Input: part model. Units: mm. Frame: model coordinates. A direction names the side the tool comes from. Give positions to 0.01 mm unless a question says otherwise; leave off trailing zeros. Order: outer loops, then holes, each group sorted by start corner. A loop starts at its lowest first (then second) coordinate and runs counter-clockwise, first axis right, second up. Notation, with made-up numbers: M -1,69 L 13,69 A9 ccw 13,77 Z; hole C 24.25,69 d6. An arc over 180 degrees is marked long. Use a Markdown table: item, result.
from build123d import *

# Parameters (mm, degrees)
F0_R     = 75
F0_R_2   = 67.5
F5_R     = 7.5
F6_DEPTH = 150


with BuildPart() as f2:
    # F2: sweep along a path in F1
    with BuildLine(Plane.XY) as f2_path:
        Line((0, 0), (0, 250))
        ThreePointArc((0, 250), (-41.0050506339, 348.9949493661), (-140, 390))
        Line((-140, 390), (-390, 390))
    # F0 (on Front) → F2 (sweep)
    with BuildSketch(Plane.XZ):
        Circle(F0_R)
        Circle(F0_R_2, mode=Mode.SUBTRACT)
    sweep(path=f2_path.line)

    # F5 (on face) → F6 (cut)
    with BuildSketch(Plane(origin=(267.132034356, 267.132034356, 0), x_dir=(-0.7071067812, 0.7071067812, 0), z_dir=(0.7071067812, 0.7071067812, 0))):
        with Locations((276.0982438922, 0)):
            Circle(F5_R)
    extrude(amount=-F6_DEPTH, mode=Mode.SUBTRACT)


solid = f2.part
1) Cut plane A-A on z = 22. Return loops of the section in (x, y).
Response values:
| item | result |
|---|---|
| outline | M -390,318.3 L -140,318.3 A68.3 cw -71.7,250 L -71.7,0 L -63.81,0 L -63.81,250 A76.19 ccw -140,326.19 L -390,326.19 Z; M -390,453.81 L -140,453.81 A203.81 cw 63.81,250 L 63.81,0 L 71.7,0 L 71.7,250 A211.7 ccw -140,461.7 L -390,461.7 Z |
2) First-contact query: pin 1 Ø2 at (x, z) = (-42.5, -37.5) entering from -Y; pin 2 Ø4 at (y, z) = (167.5, -53.5) entering from +X; pin 3 Ø2 at (y, z) = (144, -9) entering from +X. Flat tips, straight axial feed; report the tip coordinate or a pass-through.
Response values:
| item | result |
|---|---|
| pin 1 | stops at y = 419.2 |
| pin 2 | stops at x = 54.52 |
| pin 3 | stops at x = 74.57 |
3) Material intervals for line 1 (Z direction, x = -216, y = 390); line 2 (Y direction, x = -325, z = 0), sorted ascending. Write a range as from..to.
Response values:
| item | result |
|---|---|
| line 1 | z = -75..-67.5, 67.5..75 |
| line 2 | y = 315..322.5, 457.5..465 |
4) Cut plane C-C on z = -45. Return loops of the section in (x, y), and give its area (3 significant figures).
Response values:
| item | result |
|---|---|
| outline | M -390,330 L -140,330 A80 cw -60,250 L -60,0 L -50.31,0 L -50.31,250 A89.69 ccw -140,339.69 L -390,339.69 Z; M -390,440.31 L -140,440.31 A190.31 cw 50.31,250 L 50.31,0 L 60,0 L 60,250 A200 ccw -140,450 L -390,450 Z |
| area | 13,900 mm² |
5) Reachability of faces 1 (the face through (-266.75, 322.565, -2.968)), 2 (the face through (11, 0, 67)), 3 (the face through (-9.764, 126.75, -74.362)) from +Z, -Z, +X, -X, +Y, -Y: full face, straight path, thin tool, end or side. Return the list, or none.
Response values:
| item | result |
|---|---|
| face 1 | -X |
| face 2 | +Z, -Z, +X, -X, -Y |
| face 3 | -Y |
6) Mould query, pull axis Z, two halves, no side actions, for faces 4 (the face through (-390, 379, -67)), 5 (the face through (-266.75, 459.28, 28.73)), 6 (the face through (14.292, 394.157, 0.33)), 7 (the face through (-53.57, 126.75, 41.07)). Classes: released by +Z, released by -Z, zero draft, split by the parting line, or undercut.
Response values:
| item | result |
|---|---|
| face 4 | zero draft |
| face 5 | split by the parting line |
| face 6 | undercut |
| face 7 | undercut |
7) Cut plane B-B on x = -152. Return loops of the section in (y, z).
Response values:
| item | result |
|---|---|
| outline | C 390,0 d150; hole C 390,0 d135 |
